Source: CAD feature listing. Evaluate the final solid. Frame: model axes, mm. Face numbers are marked on the shaded views. Give positions to 0.01 mm unless a question says otherwise; leave off trailing zeros. Loops run counter-clockwise (first coordinate to the right, second up) from the corner with the lowest first, then second, coordinate; pieces in that order, holes last. Notation, with made-up numbers: (3.5, 74.5) - (25.5, 74.5) arc R31 ccw to (25.5, 107.5) - close; hole circle Ø7 at (88.25, -28.75). An arc over 180 degrees is marked (long way). Put each result on its own line as item: value.
```python
from build123d import *

# Parameters (mm, degrees)
CYLINDER001_R               = 4
CYLINDER001_DEPTH           = 10
CYLINDER001_PLACEMENT_ANGLE = 45
CYLINDER_R                  = 2.5
CYLINDER_DEPTH              = 10
PAD006_DEPTH                = 1


with BuildPart() as cylinder001:
    # Cylinder001 → Cylinder001 (new body)
    with BuildSketch(Plane.XY):
        Circle(CYLINDER001_R)
    extrude(amount=CYLINDER001_DEPTH)


with BuildPart() as cylinder001_1:
    # Cylinder001 placement: moved
    add(cylinder001.part.moved(Location((0, -13.435029, 5.535534))).rotate(Axis((0, -13.435029, 5.535534), (-1, 0, 0)), CYLINDER001_PLACEMENT_ANGLE))


with BuildPart() as cylinder:
    # Cylinder → Cylinder (new body)
    with BuildSketch(Plane(origin=(0, -6, 10), x_dir=(0, 0, 1), z_dir=(0, 1, 0))):
        Circle(CYLINDER_R)
    extrude(amount=CYLINDER_DEPTH)


with BuildPart() as obj1:
    # Sketch009 → Pad006 (new body, symmetric)
    with BuildSketch(Plane.XZ):
        with BuildLine():
            Line((22.524081, 18), (0.5, 2))
            Line((0.5, 2), (0, 2))
            Line((-0.5, 2), (0, 2))
            Line((-22.524081, 18), (-0.5, 2))
            ThreePointArc((-22.524081, 18), (0, 10.908086), (22.524081, 18))
        make_face()
    extrude(amount=PAD006_DEPTH, both=True)

    # Cut002: cut Cylinder
    add(cylinder.part, mode=Mode.SUBTRACT)


with BuildPart() as obj2:
    # Sketch008 → Revolution001 (revolve)
    with BuildSketch(Plane.YZ):
        Polygon((0, 2), (0, 0), (2.5, 0), (2.5, 2), (24.5, 18), (22.5, 18), (0.5, 2), align=None)
    revolve(axis=Axis((0, 0, 0), (0, 0, 1)))

    # Fusion002: union obj1
    add(obj1.part)

    # Cut003: cut Cylinder001
    add(cylinder001_1.part, mode=Mode.SUBTRACT)


with BuildPart() as obj2_1:
    # Cut003 placement: moved
    add(obj2.part.moved(Location((0, -27, -18))))


with BuildPart() as obj2_2:
    # Body009 placement: moved
    add(obj2_1.part.moved(Location((0, 50, 0))))


solid = obj2_2.part
```
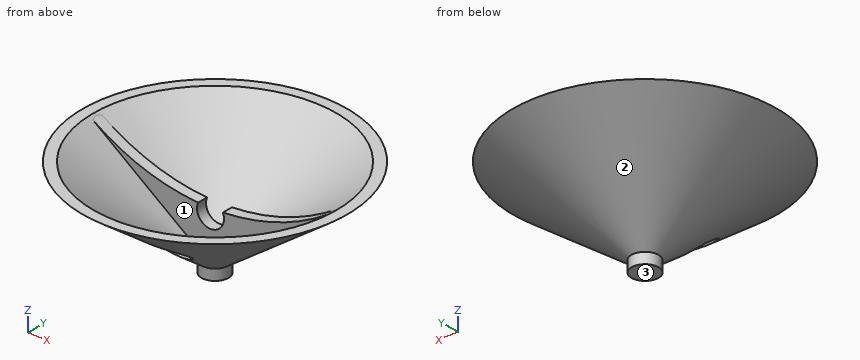
1) Section query A-A, the plane x = 0. Output: boundary loops of the cut face in (y, z).
Check result:
outline: (-1.5, 0) - (8.85, -7.53) - (9.69, -6.68) - (0.5, 0) - close; (15.4, -12.29) - (20.5, -16) - (20.5, -18) - (25.5, -18) - (25.5, -16) - (47.5, 0) - (45.5, 0) - (24, -15.64) - (24, -10.5) - (22, -10.5) - (22, -15.64) - (16.24, -11.45) - close
2) Pin query (flat end, axial travel): P1, Ø3, axis at x = -13.5, z = -3.5, coming from the -Y side; P2, Ø7.5, axis at x = 9.5, z = -11, coming from the -Y side; P3, Ø10, axis at x = 7, y = 39, coming from the -Z side; P4, Ø6, axis at y = 39, z = -12.5, coming from the +X side. Return the tip coordinate at first contact, or that it passes through.
Check result:
P1: y = 5.7
P2: y = 11.39
P3: z = -8.75
P4: through
3) Material intervals for line 1 along Y through (x, z) = (-7, -7.75); line 2 along Y through (x, z) = (7.5, -9.25); line 3 along Z through (x, y) = (0, 23.4), sorted ascending. Write a range as [from, to].
Check result:
line 1: [11.06, 13.45], [22, 24], [32.55, 34.94]
line 2: [13.91, 16.72], [22, 24], [29.28, 32.09]
line 3: [-18, -10.5]
4) Mould query, pull axis Y, two halves, no side actions, for the marked faces 1, 2 and 3. Classes: pulls with the +Y half, pulls with the -Y half, needs draft (parallel to the pull), parting line crosses it, or undercut.
Check result:
face 1: undercut
face 2: parting line crosses it
face 3: needs draft
5) Section query C-C, the plane z = -13.75. Output: boundary loops of the cut face in (x, y).
Check result:
outline: circle Ø11.19 at (0, 23); hole (-3.45, 22) arc R3.59 ccw to (3.45, 22) - close; hole (-3.45, 24) - (3.45, 24) arc R3.59 ccw to start
